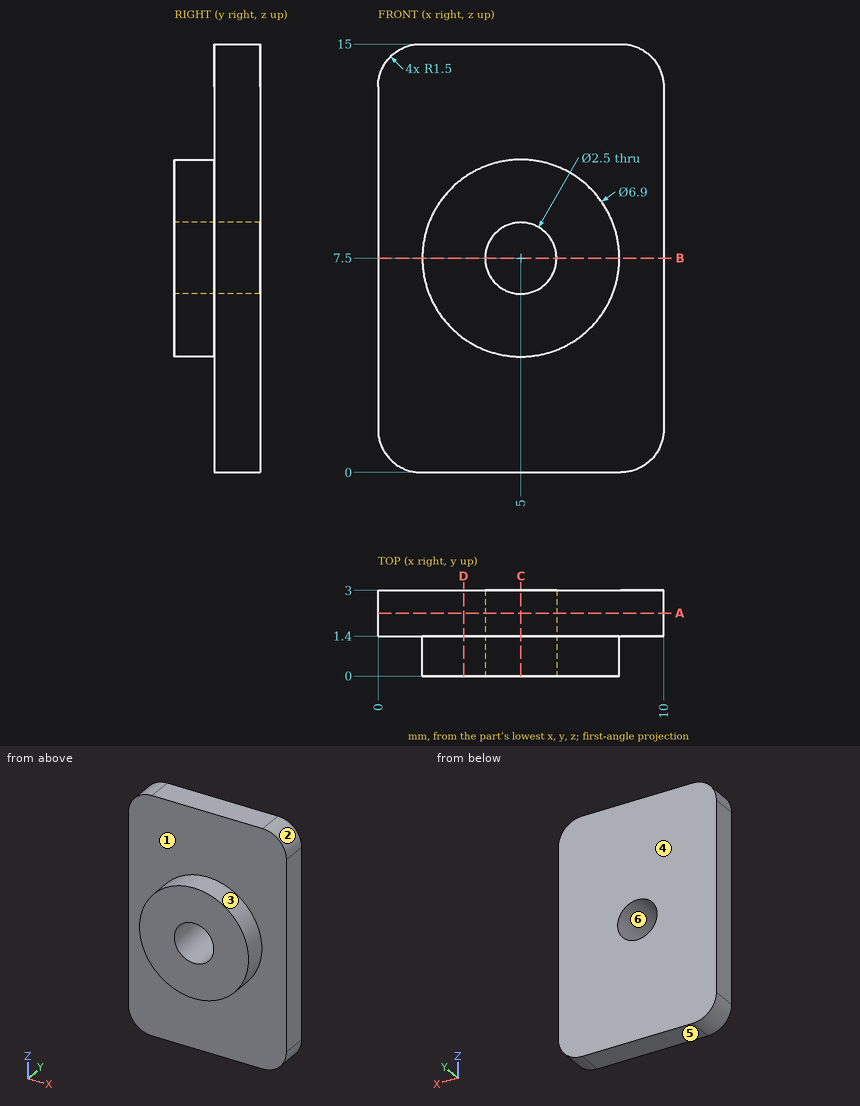
Can you work these out from the drawing? Everything is in mm from the part's minimum corner. A direction names the side the tool comes from. Coordinates: 2 decimals unless noted, no trailing zeros. Loops run counter-clockwise (first coordinate to the right, second up) from the corner with the lowest first, then second, coordinate; pieces in that order, holes last. Notation, with made-up numbers: (-25.75, 46) -> (-15.75, 46) arc R25 cw to (-15.75, 67) -> close; hole circle Ø3 at (64, 69). An arc over 180 degrees is marked (long way). Return JSON: item names as keys, results as strings.
1) If we section it at A-A, the plane y = 2.2: Write out the boundary of the cut face in (x, z).
Results below:
{"outline": "(0, 1.5) arc R1.5 ccw to (1.5, 0) -> (8.5, 0) arc R1.5 ccw to (10, 1.5) -> (10, 13.5) arc R1.5 ccw to (8.5, 15) -> (1.5, 15) arc R1.5 ccw to (0, 13.5) -> close; hole circle Ø2.5 at (5, 7.5)"}
2) If we section it at C-C, the plane x = 5: Write out the boundary of the cut face in (y, z).
Results below:
{"outline": "(0, 4.05) -> (1.4, 4.05) -> (1.4, 0) -> (3, 0) -> (3, 6.25) -> (0, 6.25) -> close; (0, 8.75) -> (3, 8.75) -> (3, 15) -> (1.4, 15) -> (1.4, 10.95) -> (0, 10.95) -> close"}
3) For the marked faces 1 and 2, which set-ups out of +Z, -Z, +X, -X, +Y, -Y let a thin tool reach every point of the face, with its end or its side?
Results below:
{"face 1": "-Y", "face 2": "+Z, +X, +Y, -Y"}
4) Will this pin go through, and if not, where does the flat tip stop? pin 1 (3 mm diameter, centred on x = 5, z = 7.5, fed in from -Y).
Results below:
{"pin 1": "y = 0"}
5) I need wall thicknesses on line 1 (Z direction, x = 5, y = 1.85); line 2 (Y direction, x = 8.25, z = 3.75); line 3 (Z direction, x = 5.25, y = 0.15). Which ranges of each line are inside material? Lowest first, please. Write a range as from..to.
Results below:
{"line 1": "0..6.25, 8.75..15", "line 2": "1.4..3", "line 3": "4.06..6.28, 8.72..10.94"}
6) Thinking about a two-plate mould opening in Z: for the marked faces 3, 4, 5 and 6, which applies, +Z half, -Z half, draft (parallel to the pull), parting line (faces both ways), or undercut?
Results below:
{"face 3": "parting line", "face 4": "draft", "face 5": "-Z half", "face 6": "undercut"}
7) If we section it at D-D, the plane x = 3: Write out the boundary of the cut face in (y, z).
Results below:
{"outline": "(0, 4.69) -> (1.4, 4.69) -> (1.4, 0) -> (3, 0) -> (3, 15) -> (1.4, 15) -> (1.4, 10.31) -> (0, 10.31) -> close"}
8) If we section it at B-B, the plane z = 7.5: Write out the boundary of the cut face in (x, y), then the cut area to 3 significant figures.
Results below:
{"outline": "(0, 1.4) -> (1.55, 1.4) -> (1.55, 0) -> (3.75, 0) -> (3.75, 3) -> (0, 3) -> close; (6.25, 0) -> (8.45, 0) -> (8.45, 1.4) -> (10, 1.4) -> (10, 3) -> (6.25, 3) -> close", "area": "18.2 mm²"}
